```python
from build123d import *

# Parameters (mm, degrees)
F1_DEPTH = 5


with BuildPart() as f1:
    # F0 (on Top) → F1 (new body)
    with BuildSketch(Plane.XY):
        with BuildLine():
            Line((-3, 0), (0, 0))
            Line((0, 0), (0, 9))
            ThreePointArc((0, 9), (-0.292893, 9.707107), (-1, 10))
            Line((-1, 10), (-10, 10))
            ThreePointArc((-10, 10), (-10.707107, 9.707107), (-11, 9))
            Line((-11, 9), (-11, -4))
            ThreePointArc((-11, -4), (-11.292893, -4.707107), (-12, -5))
            Line((-12, -5), (-15, -5))
            ThreePointArc((-15, -5), (-15.707107, -4.707107), (-16, -4))
            Line((-16, -4), (-16, 1))
            ThreePointArc((-16, 1), (-16.292893, 1.707107), (-17, 2))
            Line((-17, 2), (-18, 2))
            ThreePointArc((-18, 2), (-18.707107, 1.707107), (-19, 1))
            Line((-19, 1), (-19, -7))
            ThreePointArc((-19, -7), (-18.707107, -7.707107), (-18, -8))
            Line((-18, -8), (-11, -8))
            Line((-11, -8), (-11, -20))
            Line((-11, -20), (-7, -20))
            Line((-7, -20), (-7, 6))
            ThreePointArc((-7, 6), (-6.707107, 6.707107), (-6, 7))
            Line((-6, 7), (-4, 7))
            ThreePointArc((-4, 7), (-3.292893, 6.707107), (-3, 6))
            Line((-3, 6), (-3, 0))
        make_face()
    extrude(amount=F1_DEPTH)


solid = f1.part
```
The model under review builds one solid part; all positions refer to its coordinate system, in mm. A direction names the side the tool comes from. Round coordinates to 2 decimals unless told otherwise and drop trailing zeros. Write each loop counter-clockwise with the first axis right and the second up, starting at its lowest first coordinate (ties: lowest second). Pieces come first, ordered by that corner, then holes. Notation, with made-up numbers: (46, 49) - (80, 49) arc R19 cw to (80, 63) - close; hole circle Ø11 at (50.25, -25). An arc over 180 degrees is marked (long way). Answer as CSV lines item,"result". Start each with the question number.
(1) We need section D-D on y = 8. State the section outline as (x, z) points.
(2) For pin 1 Ø0.5 at (x, z) = (-17.5, 2) entering from +Y; pin 2 Ø1 at (y, z) = (-9.5, 3.5) entering from -X; pin 3 Ø1.5 at (y, z) = (-2, 2) entering from +X, all flat-tipped, find the tip position at first contact; note any pin that passes through.
(3) We need section C-C on x = -13.5. State the section outline as (y, z) points, plus the area to 3 significant figures.
(4) We need section A-A on y = -2. State the section outline as (x, z) points, plus the area to 3 significant figures.
(5) We need section B-B on z = 1.8. State the section outline as (x, y) points, plus the area to 3 significant figures.
(6) To check wall thickness, follow line 1 (X direction, y = 0.5, z = 2.5); line 2 (X direction, y = 6, z = 4.15); line 3 (Y direction, x = -13.5, z = 0.4). State the ranges of each line that lie inside material, in increasing order.
(7) Draft analysis for pull direction X (two halves, no side actions). For faces 1 (the cylindrical face through (-10.699, 9.715, 2.465)), 2 (the flat face through (-10, -3, 0)), 3 (the cylindrical face through (-16.285, 1.699, 2.465)), 4 (the cylindrical face through (-0.285, 9.699, 2.465)), state which applies: pulls with the +X half, pulls with the -X half, needs draft (parallel to the pull), parting line crosses it, or undercut.
(8) For faces 5 (the flat face through (-15, -8, 2)), 6 (the flat face through (-17.5, 2, 2.5)), 7 (the flat face through (-3, 3, 2)), 8 (the flat face through (-16, -2, 2)), list the 3-axis set-ups (+Z, -Z, +X, -X, +Y, -Y) from which the entire face can be reached by the end or side of a thin tool; tool diameter is ignored.
Worked answers:
1,outline,"(-11, 0) - (0, 0) - (0, 5) - (-11, 5) - close"
2,pin 1,"y = 2"
2,pin 2,"x = -11"
2,pin 3,"x = -7"
3,outline,"(-8, 0) - (-5, 0) - (-5, 5) - (-8, 5) - close"
3,area,"15.0 mm²"
4,outline,"(-19, 0) - (-16, 0) - (-16, 5) - (-19, 5) - close; (-11, 0) - (-7, 0) - (-7, 5) - (-11, 5) - close"
4,area,"35.0 mm²"
5,outline,"(-19, -7) arc R1 ccw to (-18, -8) - (-11, -8) - (-11, -20) - (-7, -20) - (-7, 6) arc R1 cw to (-6, 7) - (-4, 7) arc R1 cw to (-3, 6) - (-3, 0) - (0, 0) - (0, 9) arc R1 ccw to (-1, 10) - (-10, 10) arc R1 ccw to (-11, 9) - (-11, -4) arc R1 cw to (-12, -5) - (-15, -5) arc R1 cw to (-16, -4) - (-16, 1) arc R1 ccw to (-17, 2) - (-18, 2) arc R1 ccw to (-19, 1) - close"
5,area,"207 mm²"
6,line 1,"-19 to -16, -11 to -7, -3 to 0"
6,line 2,"-11 to -7, -3 to 0"
6,line 3,"-8 to -5"
7,face 1,"pulls with the -X half"
7,face 2,"needs draft"
7,face 3,"undercut"
7,face 4,"pulls with the +X half"
8,face 5,"+Z, -Z, -X, -Y"
8,face 6,"+Z, -Z, -X, +Y"
8,face 7,"+Z, -Z, -Y"
8,face 8,"+Z, -Z, +Y"
